Model file for the job. Use its own axes, mm. Face numbers are marked on the shaded views. A direction names the side the tool comes from. Give positions to 0.01 mm unless a question says otherwise; leave off trailing zeros. Loops run counter-clockwise (first coordinate to the right, second up) from the corner with the lowest first, then second, coordinate; pieces in that order, holes last. Notation, with made-up numbers: (59, -34) - (107, -34) arc R12 cw to (107, -12) - close; hole circle Ø9 at (33.25, 74). An arc over 180 degrees is marked (long way). Use a Markdown table: item, result.
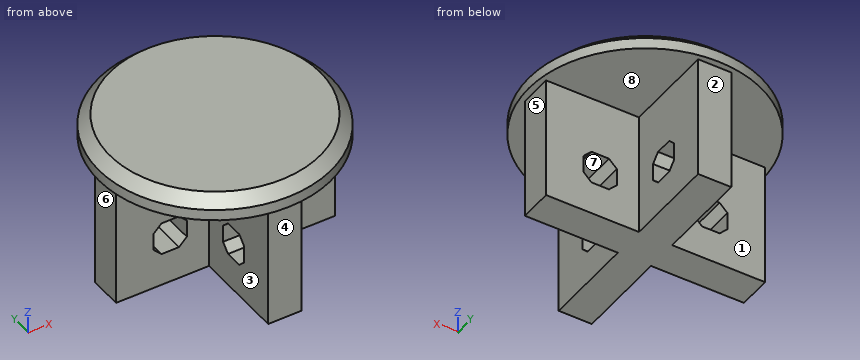
from build123d import *

# Parameters (mm, degrees)
PAD042_DEPTH    = 11.2
SKETCH075_R     = 10.5
PAD043_DEPTH    = 2
CHAMFER004_SIZE = 1
POCKET032_DEPTH = 12.001018
POCKET033_DEPTH = 12.001


with BuildPart() as part:
    # Sketch074 (on Face4 of Binder018) → Pad042 (new body)
    with BuildSketch(Plane.XY.offset(89.8)):
        Polygon((-85.13961, 93.539629), (-82.13961, 93.539629), (-82.13961, 85.139629), (-73.73961, 85.139629), (-73.73961, 82.139629), (-82.13961, 82.139592), (-82.13961, 73.739592), (-85.13961, 73.739592), (-85.13961, 82.139592), (-93.53961, 82.139592), (-93.53961, 85.139629), (-85.13961, 85.139629), align=None)
    extrude(amount=PAD042_DEPTH)

    # Sketch075 (on Face14 of Pad042) → Pad043 (join)
    with BuildSketch(Plane.XY.offset(101)):
        with Locations((-83.63961, 83.63961)):
            Circle(SKETCH075_R)
    extrude(amount=PAD043_DEPTH)

    # Chamfer004
    chamfer004_edges = [part.edges().sort_by_distance(p)[0] for p in [
        (-94.13961, 83.63961, 103),
    ]]
    chamfer(chamfer004_edges, length=CHAMFER004_SIZE)

    # Sketch076 (on Face6 of Chamfer004) → Pocket032 (cut, through all)
    with BuildSketch(Plane(origin=(0, 85.139629, 0), x_dir=(-1, 0, 0), z_dir=(0, 1, 0))):
        Polygon((77.846717, 95.8), (79.432503, 95.8), (80.13961, 95.092893), (80.13961, 93.507107), (79.432503, 92.8), (77.846717, 92.8), (77.13961, 93.507107), (77.13961, 95.092893), align=None)
        Polygon((87.13961, 95.092893), (87.846717, 95.8), (89.432504, 95.8), (90.13961, 95.092893), (90.13961, 93.507107), (89.432504, 92.8), (87.846717, 92.8), (87.13961, 93.507107), align=None)
    extrude(amount=-POCKET032_DEPTH, mode=Mode.SUBTRACT)

    # Sketch077 (on Face15 of Pocket032) → Pocket033 (cut, through all)
    with BuildSketch(Plane(origin=(-82.139609, -1e-06, 0), x_dir=(0, 1, 0), z_dir=(1, 0, 0))):
        Polygon((87.846736, 95.8), (89.432523, 95.8), (90.139629, 95.092893), (90.139629, 93.507107), (89.432523, 92.8), (87.846736, 92.8), (87.139629, 93.507107), (87.139629, 95.092893), align=None)
        Polygon((77.846699, 95.8), (79.432486, 95.8), (80.139593, 95.092893), (80.139593, 93.507107), (79.432486, 92.8), (77.846699, 92.8), (77.139593, 93.507107), (77.139593, 95.092893), align=None)
    extrude(amount=-POCKET033_DEPTH, mode=Mode.SUBTRACT)


solid = part.part
(1) 3-axis set-ups, long thin cutter, end or side, ignore diameter. For the marked faces 1, 2, 3 and 4: which of +Z, -Z, +X, -X, +Y, -Y reach the whole face in a straight line?
Computed:
| item | result |
|---|---|
| face 1 | -Z, -X, +Y |
| face 2 | -Z, +X, -X, +Y |
| face 3 | -Z, -X, -Y |
| face 4 | -Z, +X, -X, -Y |
(2) Mould opens along X. For the marked faces 5, 6, 7 and 8 say: pulls with the +X half, pulls with the -X half, needs draft (parallel to the pull), parting line crosses it, or undercut.
Computed:
| item | result |
|---|---|
| face 5 | pulls with the +X half |
| face 6 | pulls with the -X half |
| face 7 | undercut |
| face 8 | needs draft |
(3) Slice it at A-A, the plane z = 94. Write the cut outline in (x, y).
Computed:
| item | result |
|---|---|
| outline | (-93.54, 82.14) - (-90.14, 82.14) - (-90.14, 85.14) - (-93.54, 85.14) - close; (-87.14, 82.14) - (-85.14, 82.14) - (-85.14, 80.14) - (-82.14, 80.14) - (-82.14, 82.14) - (-80.14, 82.14) - (-80.14, 85.14) - (-82.14, 85.14) - (-82.14, 87.14) - (-85.14, 87.14) - (-85.14, 85.14) - (-87.14, 85.14) - close; (-85.14, 73.74) - (-82.14, 73.74) - (-82.14, 77.14) - (-85.14, 77.14) - close; (-85.14, 90.14) - (-82.14, 90.14) - (-82.14, 93.54) - (-85.14, 93.54) - close; (-77.14, 82.14) - (-73.74, 82.14) - (-73.74, 85.14) - (-77.14, 85.14) - close |
(4) Slice it at B-B, the plane z = 100.5. Write the cut outline in (x, y).
Computed:
| item | result |
|---|---|
| outline | (-93.54, 82.14) - (-85.14, 82.14) - (-85.14, 73.74) - (-82.14, 73.74) - (-82.14, 82.14) - (-73.74, 82.14) - (-73.74, 85.14) - (-82.14, 85.14) - (-82.14, 93.54) - (-85.14, 93.54) - (-85.14, 85.14) - (-93.54, 85.14) - close |
(5) Slice it at C-C, the plane x = -83. Count the separate pieces of the cut face and the enclosed holes in it, plus the area to 3 significant figures.
Computed:
| item | result |
|---|---|
| separate pieces | 1 |
| enclosed holes | 2 |
| area | 247 mm² |
(6) Drill centre lines: probe 1 along Y at (x, z) = (-83.5, 95.25); probe 2 along Y at (x, z) = (-83, 97); probe 3 along Y at (x, z) = (-86, 95.25). Where is each one in solid material? Low to high. Write a range as [from, to].
Computed:
| item | result |
|---|---|
| probe 1 | [73.74, 77.3], [79.98, 87.3], [89.98, 93.54] |
| probe 2 | [73.74, 93.54] |
| probe 3 | [82.14, 85.14] |
(7) Pin check, flat tips, straight feed: P1, Ø5, axis at y = 80.5, z = 91.5, coming from the -X side; P2, Ø6.5, axis at x = -90.5, z = 97.5, coming from the -Y side; P3, Ø1.7, axis at y = 83.5, z = 94.5, coming from the +X side. Stop position of each tip, or through.
Computed:
| item | result |
|---|---|
| P1 | x = -93.54 |
| P2 | y = 82.14 |
| P3 | x = -73.74 |
